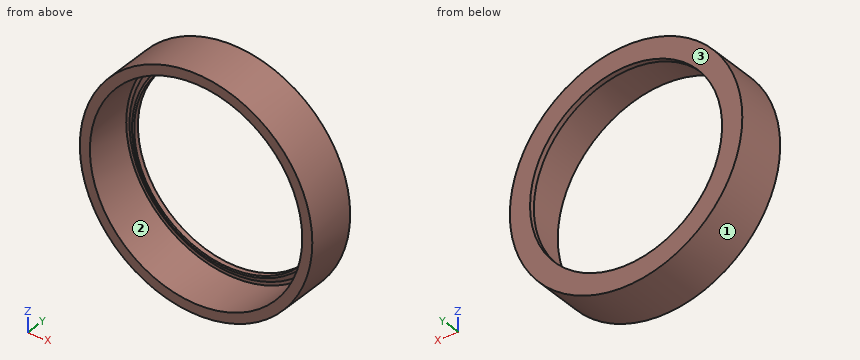
from build123d import *

# Parameters (mm, degrees)
SKETCH1_R           = 115
SKETCH1_R_2         = 105.05
BOSS_EXTRUDE1_DEPTH = 50
SKETCH2_R           = 105.05
SKETCH2_R_2         = 95
BOSS_EXTRUDE2_DEPTH = 5
SKETCH3_R           = 105.05
SKETCH3_R_2         = 101.75
CUT_EXTRUDE1_DEPTH  = 3


with BuildPart() as part:
    # Sketch1 → Boss-Extrude1 (new body)
    with BuildSketch(Plane(origin=(0, 0, 0), x_dir=(1, 0, 0), z_dir=(0, 1, 0))):
        Circle(SKETCH1_R)
        Circle(SKETCH1_R_2, mode=Mode.SUBTRACT)
    extrude(amount=BOSS_EXTRUDE1_DEPTH)

    # Sketch2 → Boss-Extrude2 (add)
    with BuildSketch(Plane(origin=(0, 50, 0), x_dir=(1, 0, 0), z_dir=(0, 1, 0))):
        Circle(SKETCH2_R)
        Circle(SKETCH2_R_2, mode=Mode.SUBTRACT)
    extrude(amount=-BOSS_EXTRUDE2_DEPTH)

    # Sketch3 → Cut-Extrude1 (cut)
    with BuildSketch(Plane.XZ.offset(-45)):
        Circle(SKETCH3_R)
        Circle(SKETCH3_R_2, mode=Mode.SUBTRACT)
    extrude(amount=-CUT_EXTRUDE1_DEPTH, mode=Mode.SUBTRACT)

    # Sketch6 → Cut-Revolve1 (revolve, cut)
    with BuildSketch(Plane.XY):
        Polygon((102, 48), (97, 45), (102, 45), align=None)
    revolve(axis=Axis((0, 48, 0), (0, -1, 0)), mode=Mode.SUBTRACT)


solid = part.part
Part model, mm, in its own coordinate system. Face numbers are marked on the shaded views. Coordinates: 2 decimals unless noted, no trailing zeros. Loops run counter-clockwise (first coordinate to the right, second up) from the corner with the lowest first, then second, coordinate; pieces in that order, holes last. Notation, with made-up numbers: M 47.5,14 L 66.5,14 A15 ccw 66.5,33 Z; hole C 84,1.5 d7. An arc over 180 degrees is marked long. Use a Markdown table: item, result. Add a question column.
Q1. Mould opens along X. For the marked faces 1, 2 and 3 say: +X half, -X half, draft (parallel to the pull), parting line (faces both ways), or undercut.
Q2. Cut at C-C (y = 31.5). Write the cut outline in (x, z).
Q3. Pin check, flat tips, straight feed: P1, Ø5, axis at y = 36.5, z = 14, coming from the -X side; P2, Ø2, axis at y = 38, z = -58, coming from the -X side; P3, Ø10, axis at x = 16.5, y = 28, coming from the +Z side. Stop position of each tip, or through.
Q4. Probe L1, parallel to Z at x = 0, y = 15; L2, parallel to Z at x = 0, y = 47.55. List the from-to ranges inside material, lowest first.
Q5. Cut at B-B (z = 0). Write the cut outline in (x, y), and give its area (3 significant figures).
Q6. Cut at A-A (x = 0). Write the cut outline in (y, z).
Worked out:
| question | item | result |
|---|---|---|
| 1 | face 1 | parting line |
| 1 | face 2 | undercut |
| 1 | face 3 | draft |
| 2 | outline | C 0,0 d230; hole C 0,0 d210.1 |
| 3 | P1 | stops at x = -114.42 |
| 3 | P2 | stops at x = -99.88 |
| 3 | P3 | stops at z = 114.42 |
| 4 | L1 | z = -115 to -105.05, 105.05 to 115 |
| 4 | L2 | z = -115 to -105.05, -101.25 to -95, 95 to 101.25, 105.05 to 115 |
| 5 | outline | M -115,0 L -105.05,0 L -105.05,48 L -101.75,48 L -101.75,47.85 L -97,45 L -95,45 L -95,50 L -115,50 Z; M 95,45 L 97,45 L 101.75,47.85 L 101.75,48 L 105.05,48 L 105.05,0 L 115,0 L 115,50 L 95,50 Z |
| 5 | area | 1,060 mm2 |
| 6 | outline | M 0,-115 L 50,-115 L 50,-95 L 45,-95 L 45,-97 L 47.85,-101.75 L 48,-101.75 L 48,-105.05 L 0,-105.05 Z; M 0,105.05 L 48,105.05 L 48,101.75 L 47.85,101.75 L 45,97 L 45,95 L 50,95 L 50,115 L 0,115 Z |
